```python
from build123d import *

# Parameters (mm, degrees)
SKETCH1_R           = 3
BOSS_EXTRUDE1_DEPTH = 5
FILLET1_R           = 1


with BuildPart() as part:
    # Sketch1 → Boss-Extrude1 (new body)
    with BuildSketch(Plane.XY):
        with BuildLine():
            Line((-7.217785759, 14.139278402), (-6.99958338, 34.13808806))
            ThreePointArc((-6.99958338, 34.13808806), (0, 41.061717228), (6.99958338, 34.13808806))
            Line((6.99958338, 34.13808806), (7.217785759, 14.139278402))
            ThreePointArc((7.217785759, 14.139278402), (0, 15.875), (-7.217785759, 14.139278402))
        make_face()
        with Locations((0, 34.061717228)):
            Circle(SKETCH1_R, mode=Mode.SUBTRACT)
    extrude(amount=BOSS_EXTRUDE1_DEPTH)

    # Fillet1
    fillet1_edges = [part.edges().sort_by_distance(p)[0] for p in [
        (-7.217785759, 14.139278402, 2.5),
        (7.217785759, 14.139278402, 2.5),
    ]]
    fillet(fillet1_edges, radius=FILLET1_R)


solid = part.part
```
Could you check a few things on this model? Use its own coordinates, in mm. Coordinates: 2 decimals unless noted, no trailing zeros. Loops run counter-clockwise (first coordinate to the right, second up) from the corner with the lowest first, then second, coordinate; pieces in that order, holes last.
1) Will these pins go through, and if not, where does the flat tip stop? pin 1 Ø1.5 at (y, z) = (21, 2) entering from -X; pin 2 Ø1 at (x, z) = (-5, 3) entering from -Y.
Reported:
pin 1: stops at x = -7.15
pin 2: stops at y = 14.89
2) Please list where these lines run through material, in increasing order: line 1 along Y through (x, z) = (2.5, 0.6); line 2 along Y through (x, z) = (-2, 2.45); line 3 along X through (y, z) = (33.75, 4.3).
Reported:
line 1: y = 15.68 to 32.4, 35.72 to 40.6
line 2: y = 15.75 to 31.83, 36.3 to 40.77
line 3: x = -7 to -2.98, 2.98 to 7
3) Imagine slicing it at A-A (x = 0). List the corners of the cut face in (y, z) for me (3 decimals), and give its area (3 significant figures).
Reported:
outline: (15.875, 0) - (31.062, 0) - (31.062, 5) - (15.875, 5) - close; (37.062, 0) - (41.062, 0) - (41.062, 5) - (37.062, 5) - close
area: 95.9 mm2
4) Imagine slicing it at C-C (x = -4). List the corners of the cut face in (y, z) for me, and give its area (3 significant figures).
Reported:
outline: (15.36, 0) - (39.81, 0) - (39.81, 5) - (15.36, 5) - close
area: 122 mm2
5) Thinking about a two-plate mould opening in X: for faces 1 (the face through (0, 28, 0)), 2 (the face through (0.084, 15.875, 2.465)), 3 (the face through (-0.15, 41.06, 2.46)), 4 (the face through (-0.65, 31.133, 2.465)), which applies, released by +X, released by -X, zero draft, split by the parting line, or undercut?
Reported:
face 1: zero draft
face 2: undercut
face 3: split by the parting line
face 4: undercut
